from build123d import *

# Parameters (mm, degrees)
ESBO_O1_R                                      = 11
RESSALTO_EXTRUS_O1_DEPTH                       = 2.5
ESBO_O3_R                                      = 1.835521505
CORTE_EXTRUS_O1_DEPTH                          = 2.5
ESBO_O18_R                                     = 5
RESSALTO_EXTRUS_O5_DEPTH                       = 2.5
ESBO_O20_R                                     = 2
CORTE_EXTRUS_O5_DEPTH                          = 5.5
BROCA_DE_ROSQUEAR_PARA_TARRAXA_DE_M2X0_4_REACH = 21.785
BROCA_DE_ROSQUEAR_PARA_TARRAXA_DE_M2_2_R       = 0.8
ESBO_O22_R                                     = 3
CORTE_EXTRUS_O6_DEPTH                          = 5.5
ESBO_O23_R                                     = 3
CORTE_EXTRUS_O7_DEPTH                          = 1.5


with BuildPart() as part:
    # Esboço1 → Ressalto-extrusão1 (new body)
    with BuildSketch(Plane(origin=(0, 0, 0), x_dir=(1, 0, 0), z_dir=(0, 1, 0))):
        with Locations(Location((0, 0, 0), (0, 0, 270))):
            Circle(ESBO_O1_R)
    extrude(amount=RESSALTO_EXTRUS_O1_DEPTH)

    # Esboço3 → Corte-extrusão1 (cut)
    with BuildSketch(Plane(origin=(0, 2.5, 0), x_dir=(1, 0, 0), z_dir=(0, 1, 0))):
        with Locations(Location((0, 7.7, 0), (0, 0, 270))):
            Circle(ESBO_O3_R)
        with Locations(Location((6.668395609, -3.85, 0), (0, 0, 270))):
            Circle(ESBO_O3_R)
        with Locations(Location((-6.668395609, -3.85, 0), (0, 0, 270))):
            Circle(ESBO_O3_R)
    extrude(amount=-CORTE_EXTRUS_O1_DEPTH, mode=Mode.SUBTRACT)

    # Esboço18 → Ressalto-extrusão5 (add)
    with BuildSketch(Plane(origin=(0, 2.5, 0), x_dir=(1, 0, 0), z_dir=(0, 1, 0))):
        with Locations(Location((0, 0, 0), (0, 0, 270))):
            Circle(ESBO_O18_R)
    extrude(amount=RESSALTO_EXTRUS_O5_DEPTH)

    # Esboço20 → Corte-extrusão5 (cut)
    with BuildSketch(Plane(origin=(0, 5, 0), x_dir=(1, 0, 0), z_dir=(0, 1, 0))):
        with Locations(Location((0, 0, 0), (0, 0, 270))):
            Circle(ESBO_O20_R)
    extrude(amount=-CORTE_EXTRUS_O5_DEPTH, mode=Mode.SUBTRACT)

    # Broca de rosquear para tarraxa de M2 2 (on position points) → Broca de rosquear para tarraxa de M2x0.41 (cut, up to next)
    with BuildSketch(Plane(origin=(0.002598781, 3.792959438, -4.999999325), x_dir=(-0.999999864927, 0, -0.000519756122), z_dir=(0.000519756122, 0, -0.999999864927)), mode=Mode.PRIVATE) as broca_de_rosquear_para_tarraxa_de_m2x0_4_sk1:
        Circle(BROCA_DE_ROSQUEAR_PARA_TARRAXA_DE_M2_2_R)
    broca_de_rosquear_para_tarraxa_de_m2x0_4_tool1 = extrude(broca_de_rosquear_para_tarraxa_de_m2x0_4_sk1.sketch, amount=-BROCA_DE_ROSQUEAR_PARA_TARRAXA_DE_M2X0_4_REACH, mode=Mode.PRIVATE) & part.part
    add(broca_de_rosquear_para_tarraxa_de_m2x0_4_tool1.solids().sort_by_distance((0.002599, 3.792959, -4.999999))[0], mode=Mode.SUBTRACT)

    # Esboço22 → Corte-extrusão6 (cut)
    with BuildSketch(Plane(origin=(0, 2.5, 0), x_dir=(1, 0, 0), z_dir=(0, 1, 0))):
        with Locations((-11.258330249, 6.5)):
            Circle(ESBO_O22_R)
        with Locations((0, -13)):
            Circle(ESBO_O22_R)
        with Locations((11.258330249, 6.5)):
            Circle(ESBO_O22_R)
    extrude(amount=-CORTE_EXTRUS_O6_DEPTH, mode=Mode.SUBTRACT)

    # Esboço23 → Corte-extrusão7 (cut)
    with BuildSketch(Plane(origin=(0, 0, 0), x_dir=(-1, 0, 0), z_dir=(0, -1, 0))):
        with Locations(Location((-6.668395609, -3.85, 0), (0, 0, 90))):
            Circle(ESBO_O23_R)
        with Locations(Location((6.668395609, -3.85, 0), (0, 0, 90))):
            Circle(ESBO_O23_R)
        with Locations(Location((0, 7.7, 0), (0, 0, 90))):
            Circle(ESBO_O23_R)
    extrude(amount=-CORTE_EXTRUS_O7_DEPTH, mode=Mode.SUBTRACT)


solid = part.part
The model under review builds one solid part; all positions refer to its coordinate system, in mm. A direction names the side the tool comes from. Round coordinates to 2 decimals unless told otherwise and drop trailing zeros. Loops run counter-clockwise (first coordinate to the right, second up) from the corner with the lowest first, then second, coordinate; pieces in that order, holes last. Notation, with made-up numbers: M 63.5,16 L 114.5,16 A20 ccw 114.5,39 Z; hole C -20,73.25 d7. An arc over 180 degrees is marked long. Answer as a JSON object with one key per item and string values.
Item 1: We need section B-B, the plane z = 3.85. State the section outline as (x, y) points.
Check sheet entries:
{"outline": "M -10.3,0 L -9.67,0 L -9.67,1.5 L -8.5,1.5 L -8.5,2.5 L -10.3,2.5 Z; M -4.83,1.5 L -3.67,1.5 L -3.67,0 L 3.67,0 L 3.67,1.5 L 4.83,1.5 L 4.83,2.5 L 3.19,2.5 L 3.19,5 L -3.19,5 L -3.19,2.5 L -4.83,2.5 Z; M 8.5,1.5 L 9.67,1.5 L 9.67,0 L 10.3,0 L 10.3,2.5 L 8.5,2.5 Z"}
Item 2: We need section A-A, the plane z = 0. State the section outline as (x, y) points.
Check sheet entries:
{"outline": "M -11,0 L -2,0 L -2,5 L -5,5 L -5,2.5 L -11,2.5 Z; M 2,0 L 11,0 L 11,2.5 L 5,2.5 L 5,5 L 2,5 Z"}
Item 3: For line 1 along X through (y, z) = (1.7, 3.85); line 2 along X through (y, z) = (2.35, 4.5); line 3 along Z through (x, y) = (0, 3.2), list the stretches that pass through material, from the lowest coordinate up.
Check sheet entries:
{"line 1": "-10.3 to -8.5, -4.83 to 4.83, 8.5 to 10.3", "line 2": "-10.04 to -8.38, -4.95 to 4.95, 8.38 to 10.04", "line 3": "2 to 5"}
Item 4: The part is to be moulded in two halves that separate along Z. For faces 1 (the face through (-9, 1.5, 4)), 2 (the face through (0.2, 0, 2.2)), 3 (the face through (-9.592, 1.232, 5.385)), say which applies: +Z half, -Z half, draft (parallel to the pull), parting line (faces both ways), or undercut.
Check sheet entries:
{"face 1": "undercut", "face 2": "draft", "face 3": "parting line"}
Item 5: Clearance check with flat-ended pins moving along their axes: P1, Ø4, axis at x = 6.67, z = 3.85, coming from the +Y side; P2, Ø5, axis at x = 6.5, z = 3.5, coming from the -Y side. State where each tip first meets the part, or that it passes through.
Check sheet entries:
{"P1": "y = 2.5", "P2": "y = 1.5"}
Item 6: We need section C-C, the plane x = 0. State how many separate pieces and enclosed holes the cut face has, and give its area (3 significant figures).
Check sheet entries:
{"separate pieces": "4", "enclosed holes": "0", "area": "40.0 mm2"}
Item 7: We need section D-D, the plane y = 1.9. State the section outline as (x, z) points.
Check sheet entries:
{"outline": "M -10.38,-3.63 A3 cw -8.34,-7.18 A11 ccw 8.34,-7.18 A3 cw 10.38,-3.63 A11 ccw 2.05,10.81 A3 cw -2.05,10.81 A11 ccw Z; hole C -6.67,3.85 d3.67; hole C 0,0 d4; hole C 0,-7.7 d3.67; hole C 6.67,3.85 d3.67"}
Item 8: Tool access review of faces 4 (the face through (-2, 1.5, -8)), 5 (the face through (3, 2.5, 5)), 6 (the face through (0, 1, -11)), 7 (the face through (0.081, 2.007, -9.534)): name each direction out of +Z, -Z, +X, -X, +Y, -Y from which nothing blocks a thin tool from reaching the whole face with its end or side.
Check sheet entries:
{"face 4": "-Y", "face 5": "+Y", "face 6": "-Z, +Y, -Y", "face 7": "+Y, -Y"}
